Part model, mm, in its own coordinate system. Face numbers are marked on the shaded views. A direction names the side the tool comes from. Coordinates: 2 decimals unless noted, no trailing zeros. Order: outer loops, then holes, each group sorted by start corner. A loop starts at its lowest first (then second) coordinate and runs counter-clockwise, first axis right, second up. Notation, with made-up numbers: M -37,72 L 8,72 A13 cw 8,94 Z; hole C -21.75,52.25 d4. An arc over 180 degrees is marked long. Write item = value, one per line. Start each with the question number.
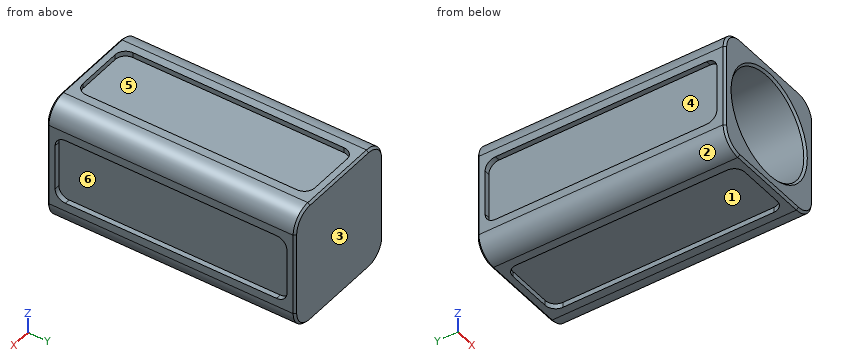
from build123d import *

# Parameters (mm, degrees)
BOSS_EXTRUDE1_DEPTH = 20
SKETCH1_3_R         = 25
BOSS_EXTRUDE2_DEPTH = 100
CUT_EXTRUDE1_DEPTH  = 2.5
CIRPATTERN1_COUNT   = 4
CHAMFER1_SIZE       = 1


with BuildPart() as part:
    # Sketch1 → Boss-Extrude1 (new body)
    with BuildSketch(Plane(origin=(0, 0, 0), x_dir=(1, 0, 0), z_dir=(0, 1, 0))):
        with BuildLine():
            Line((-65.280898876, -14.157303371), (-25.280898876, -14.157303371))
            ThreePointArc((-25.280898876, -14.157303371), (-18.209831065, -11.228371183), (-15.280898876, -4.157303371))
            Line((-15.280898876, -4.157303371), (-15.280898876, 35.842696629))
            ThreePointArc((-15.280898876, 35.842696629), (-18.209831065, 42.913764441), (-25.280898876, 45.842696629))
            Line((-25.280898876, 45.842696629), (-65.280898876, 45.842696629))
            ThreePointArc((-65.280898876, 45.842696629), (-72.351966688, 42.913764441), (-75.280898876, 35.842696629))
            Line((-75.280898876, 35.842696629), (-75.280898876, -4.157303371))
            ThreePointArc((-75.280898876, -4.157303371), (-72.351966688, -11.228371183), (-65.280898876, -14.157303371))
        make_face()
    extrude(amount=BOSS_EXTRUDE1_DEPTH)

    # Sketch1_3 → Boss-Extrude2 (add)
    with BuildSketch(Plane(origin=(0, 0, 0), x_dir=(1, 0, 0), z_dir=(0, 1, 0))):
        with BuildLine():
            Line((-65.280898876, -14.157303371), (-25.280898876, -14.157303371))
            ThreePointArc((-25.280898876, -14.157303371), (-18.209831065, -11.228371183), (-15.280898876, -4.157303371))
            Line((-15.280898876, -4.157303371), (-15.280898876, 35.842696629))
            ThreePointArc((-15.280898876, 35.842696629), (-18.209831065, 42.913764441), (-25.280898876, 45.842696629))
            Line((-25.280898876, 45.842696629), (-65.280898876, 45.842696629))
            ThreePointArc((-65.280898876, 45.842696629), (-72.351966688, 42.913764441), (-75.280898876, 35.842696629))
            Line((-75.280898876, 35.842696629), (-75.280898876, -4.157303371))
            ThreePointArc((-75.280898876, -4.157303371), (-72.351966688, -11.228371183), (-65.280898876, -14.157303371))
        make_face()
        with Locations((-45.280898876, 15.842696629)):
            Circle(SKETCH1_3_R, mode=Mode.SUBTRACT)
    extrude(amount=-BOSS_EXTRUDE2_DEPTH)

    # Sketch2 → Cut-Extrude1 (cut)
    with BuildSketch(Plane(origin=(0, 0, -45.842696629), x_dir=(-1, 0, 0), z_dir=(0, 0, -1))):
        with BuildLine():
            Line((61.280898876, -91), (61.280898876, 11))
            ThreePointArc((61.280898876, 11), (59.816432782, 14.535533906), (56.280898876, 16))
            Line((56.280898876, 16), (34.280898876, 16))
            ThreePointArc((34.280898876, 16), (30.74536497, 14.535533906), (29.280898876, 11))
            Line((29.280898876, 11), (29.280898876, -91))
            ThreePointArc((29.280898876, -91), (30.74536497, -94.535533906), (34.280898876, -96))
            Line((34.280898876, -96), (56.280898876, -96))
            ThreePointArc((56.280898876, -96), (59.816432782, -94.535533906), (61.280898876, -91))
        make_face()
    cut_extrude1 = extrude(amount=-CUT_EXTRUDE1_DEPTH, mode=Mode.SUBTRACT)

    # CirPattern1: Cut-Extrude1 ×4 about axis
    cirpattern1_axis = Axis((-45.280898876, 0, -15.842696629), (0, 1, 0))
    for i in range(1, CIRPATTERN1_COUNT):
        add(cut_extrude1.rotate(cirpattern1_axis, i * 360 / CIRPATTERN1_COUNT), mode=Mode.SUBTRACT)

    # Chamfer1
    chamfer1_edges = [part.edges().sort_by_distance(p)[0] for p in [
        (-72.351966688, 20, -42.913764441),
        (-45.280898876, 20, -45.842696629),
        (-18.209831065, 20, -42.913764441),
        (-15.280898876, 20, -15.842696629),
        (-72.351966688, -100, 11.228371183),
        (-75.280898876, -100, -15.842696629),
        (-72.351966688, -100, -42.913764441),
        (-45.280898876, -100, -45.842696629),
        (-18.209831065, -100, -42.913764441),
        (-15.280898876, -100, -15.842696629),
        (-18.209831065, -100, 11.228371183),
        (-45.280898876, -100, 14.157303371),
        (-18.209831065, 20, 11.228371183),
        (-70.280898876, -100, -15.842696629),
        (-45.280898876, 20, 14.157303371),
        (-72.351966688, 20, 11.228371183),
        (-75.280898876, 20, -15.842696629),
    ]]
    chamfer(chamfer1_edges, length=CHAMFER1_SIZE)


solid = part.part
Item 1: 3-axis set-ups, long thin cutter, end or side, ignore diameter. For the marked faces 4, 5 and 6: which of +Z, -Z, +X, -X, +Y, -Y reach the whole face in a straight line?
Item 2: Cut at A-A, the plane y = -40. Write the cut outline in (x, z).
Item 3: Wall check: line 1 along X through (y, z) = (-91.5, -15.5); line 2 along Z through (x, y) = (-46, -37); line 3 along Y through (x, z) = (-42.5, -15). Give the ranges that are in metal, low to high. Write a range as [from, to].
Item 4: Flat gauge pins, fed straight in: pin 1 (12 mm diameter, centred on y = -42.5, z = -18, fed in from -X); pin 2 (16 mm diameter, centred on x = -44, y = -42, fed in from +Z); pin 3 (3 mm diameter, centred on x = -74, y = -30.5, fed in from +Z); pin 4 (0.8 mm diameter, centred on x = -47, z = -45, fed in from +Y). Where does each tip first touch, or does it go through?
Item 5: Pull direction X, two halves, no side cores. Call the marked faces 1, 2 and 3: pulls with the +X half, pulls with the -X half, needs draft (parallel to the pull), parting line crosses it, or undercut.
Item 6: Cut at B-B, the plane y = 5.5. Write the cut outline in (x, z).
Filled sheet:
q1.face_4 = -X
q1.face_5 = +Z
q1.face_6 = +X
q2.outline = M -75.28,-35.84 A10 ccw -65.28,-45.84 L -61.28,-45.84 L -61.28,-43.34 L -29.28,-43.34 L -29.28,-45.84 L -25.28,-45.84 A10 ccw -15.28,-35.84 L -15.28,-31.84 L -17.78,-31.84 L -17.78,0.16 L -15.28,0.16 L -15.28,4.16 A10 ccw -25.28,14.16 L -29.28,14.16 L -29.28,11.66 L -61.28,11.66 L -61.28,14.16 L -65.28,14.16 A10 ccw -75.28,4.16 L -75.28,0.16 L -72.78,0.16 L -72.78,-31.84 L -75.28,-31.84 Z; hole C -45.28,-15.84 d50
q3.line_1 = [-72.78, -70.28], [-20.28, -17.78]
q3.line_2 = [-43.34, -40.83], [9.15, 11.66]
q3.line_3 = [0, 20]
q4.pin_1 = -72.78
q4.pin_2 = 11.66
q4.pin_3 = 11.08
q4.pin_4 = 20
q5.face_1 = undercut
q5.face_2 = pulls with the -X half
q5.face_3 = needs draft
q6.outline = M -75.28,-35.84 A10 ccw -65.28,-45.84 L -61.28,-45.84 L -61.28,-43.34 L -29.28,-43.34 L -29.28,-45.84 L -25.28,-45.84 A10 ccw -15.28,-35.84 L -15.28,-31.84 L -17.78,-31.84 L -17.78,0.16 L -15.28,0.16 L -15.28,4.16 A10 ccw -25.28,14.16 L -29.28,14.16 L -29.28,11.66 L -61.28,11.66 L -61.28,14.16 L -65.28,14.16 A10 ccw -75.28,4.16 L -75.28,0.16 L -72.78,0.16 L -72.78,-31.84 L -75.28,-31.84 Z
